Can you work these out from the model? Positions are in its coordinate system, mm. A direction names the side the tool comes from. Give positions to 0.01 mm unless a question says otherwise; leave off trailing zeros. Order: outer loops, then holes, each group sorted by start corner. A loop starts at its lowest first (then second) coordinate and runs counter-clockwise, first axis right, second up. Notation, with made-up numbers: (75.25, 72) - (99.25, 72) arc R25 cw to (99.25, 110) - close; hole circle Ø5 at (43, -38). An arc over 180 degrees is marked (long way). Return JSON: item names as keys, results as strings.
```python
from build123d import *

# Parameters (mm, degrees)
F0_R     = 11.08
F1_DEPTH = 7


with BuildPart() as f1:
    # F0 (on Front) → F1 (new body)
    with BuildSketch(Plane.XZ):
        with BuildLine():
            ThreePointArc((16.28, 11.08), (0.1, 15.044414), (-16.08, 11.08))
            Line((-16.08, 11.08), (-16.28, 11.08))
            ThreePointArc((-16.28, 11.08), (-18.851964, 11.455326), (-21.209412, 12.55))
            ThreePointArc((-21.209412, 12.55), (-44.425098, 0), (-21.209412, -12.55))
            ThreePointArc((-21.209412, -12.55), (-18.851964, -11.455326), (-16.28, -11.08))
            Line((-16.28, -11.08), (-16.08, -11.08))
            ThreePointArc((-16.08, -11.08), (0.1, -15.044414), (16.28, -11.08))
            ThreePointArc((16.28, -11.08), (18.851964, -11.455326), (21.209412, -12.55))
            ThreePointArc((21.209412, -12.55), (44.425098, 0), (21.209412, 12.55))
            ThreePointArc((21.209412, 12.55), (18.851964, 11.455326), (16.28, 11.08))
        make_face()
        with Locations((-29.425098, 0)):
            Circle(F0_R, mode=Mode.SUBTRACT)
        Circle(F0_R, mode=Mode.SUBTRACT)
        with Locations((29.425098, 0)):
            Circle(F0_R, mode=Mode.SUBTRACT)
    extrude(amount=F1_DEPTH)


solid = f1.part
```
1. Suppose I cut it at B-B (y = -5.5). List the corners of the cut face in (x, z) for me.
Checks:
{"outline": "(-21.21, -12.55) arc R9 cw to (-16.28, -11.08) - (-16.08, -11.08) arc R35 ccw to (16.28, -11.08) arc R9 cw to (21.21, -12.55) arc R15 ccw (long way) to (21.21, 12.55) arc R9 cw to (16.28, 11.08) arc R35 ccw to (-16.08, 11.08) - (-16.28, 11.08) arc R9 cw to (-21.21, 12.55) arc R15 ccw (long way) to start; hole circle Ø22.16 at (-29.43, 0); hole circle Ø22.16 at (0, 0); hole circle Ø22.16 at (29.43, 0)"}
2. For pin 1 Ø6 at (x, z) = (-32.5, 8.5) entering from -Y; pin 2 Ø4 at (y, z) = (-4, 8) entering from -X; pin 3 Ø1 at (x, y) = (32.5, -3.5) entering from -Z, each with a flat end and sliding along its axis, tell me the tip position at first contact or that it passes through.
Checks:
{"pin 1": "y = -7", "pin 2": "x = -43.17", "pin 3": "z = -14.78"}
3. Suppose I cut it at C-C (x = 0). List the corners of the cut face in (y, z) for me.
Checks:
{"outline": "(-7, -15.04) - (0, -15.04) - (0, -11.08) - (-7, -11.08) - close; (-7, 11.08) - (0, 11.08) - (0, 15.04) - (-7, 15.04) - close"}
4. If I drill on L1, parallel to Z at x = -30, y = -3; L2, parallel to X at y = -0.25, z = -2; L3, parallel to X at y = -6, z = -1, over which ranges is the centre line in solid material (lowest first)? Write a range as [from, to].
Checks:
{"L1": "[-14.99, -11.07], [11.07, 14.99]", "L2": "[-44.29, -40.32], [-18.53, -10.9], [10.9, 18.53], [40.32, 44.29]", "L3": "[-44.39, -40.46], [-18.39, -11.03], [11.03, 18.39], [40.46, 44.39]"}
5. Suppose I cut it at A-A (z = 0). List the corners of the cut face in (x, y) for me.
Checks:
{"outline": "(-44.43, -7) - (-40.51, -7) - (-40.51, 0) - (-44.43, 0) - close; (-18.35, -7) - (-11.08, -7) - (-11.08, 0) - (-18.35, 0) - close; (11.08, -7) - (18.35, -7) - (18.35, 0) - (11.08, 0) - close; (40.51, -7) - (44.43, -7) - (44.43, 0) - (40.51, 0) - close"}
6. Thinking about a two-plate mould opening in X: for faces 4 (the face through (-18.817, -3.451, 11.445)), 5 (the face through (10.568, -3.451, 3.328)), 6 (the face through (-10, 0, -6)), which applies, +X half, -X half, draft (parallel to the pull), parting line (faces both ways), or undercut?
Checks:
{"face 4": "undercut", "face 5": "undercut", "face 6": "draft"}
7. Suppose I cut it at D-D (z = 5). List the corners of the cut face in (x, y) for me, plus the area to 3 significant figures.
Checks:
{"outline": "(-43.57, -7) - (-39.31, -7) - (-39.31, 0) - (-43.57, 0) - close; (-19.54, -7) - (-9.89, -7) - (-9.89, 0) - (-19.54, 0) - close; (9.89, -7) - (19.54, -7) - (19.54, 0) - (9.89, 0) - close; (39.31, -7) - (43.57, -7) - (43.57, 0) - (39.31, 0) - close", "area": "195 mm^2"}
8. On a 3-axis mill with a long thin cutter (end or side, diameter ignored), from which of +Z, -Z, +X, -X, +Y, -Y can I reach the whole of each face in a straight line? I mean faces 1 (the face through (-18.887, -3.451, -11.466)), 2 (the face through (-10, -7, -6)), 3 (the face through (18.887, -3.451, 11.466)). Say none if no direction works.
Checks:
{"face 1": "-Z, +Y, -Y", "face 2": "+Z, -Z, +X, -X, -Y", "face 3": "+Z, +Y, -Y"}
